Build history of the part. All positions in model axes, mm. Give positions to 0.01 mm unless a question says otherwise; leave off trailing zeros. Write each loop counter-clockwise with the first axis right and the second up, starting at its lowest first coordinate (ties: lowest second). Pieces come first, ordered by that corner, then holes.
from build123d import *

# Parameters (mm, degrees)
SKETCH_1_W      = 72
SKETCH_1_H      = 70
SKETCH_1_R      = 2
SKETCH_1_W_2    = 40
SKETCH_1_H_2    = 40
EXTRUDE_1_DEPTH = 3
CHAMFER_1_SIZE  = 10
CHAMFER_2_SIZE  = 5


with BuildPart() as part:
    # 草图1 → 凸台-拉伸1 (new body)
    with BuildSketch(Plane(origin=(0, 0, 0), x_dir=(1, 0, 0), z_dir=(0, 1, 0))):
        Rectangle(SKETCH_1_W, SKETCH_1_H)
        with Locations(Location((-30, 30, 0), (0, 0, 270))):
            Circle(SKETCH_1_R, mode=Mode.SUBTRACT)
        with Locations(Location((30, 30, 0), (0, 0, 270))):
            Circle(SKETCH_1_R, mode=Mode.SUBTRACT)
        with Locations(Location((30, -30, 0), (0, 0, 270))):
            Circle(SKETCH_1_R, mode=Mode.SUBTRACT)
        with Locations(Location((-30, -30, 0), (0, 0, 270))):
            Circle(SKETCH_1_R, mode=Mode.SUBTRACT)
        Rectangle(SKETCH_1_W_2, SKETCH_1_H_2, mode=Mode.SUBTRACT)
    extrude(amount=EXTRUDE_1_DEPTH)

    # 倒角1
    chamfer_1_edges = [part.edges().sort_by_distance(p)[0] for p in [
        (20, 1.5, -20),
        (-20, 1.5, -20),
        (-20, 1.5, 20),
        (20, 1.5, 20),
    ]]
    chamfer(chamfer_1_edges, length=CHAMFER_1_SIZE)

    # 倒角2
    chamfer_2_edges = [part.edges().sort_by_distance(p)[0] for p in [
        (-36, 1.5, 35),
        (-36, 1.5, -35),
        (36, 1.5, -35),
        (36, 1.5, 35),
    ]]
    chamfer(chamfer_2_edges, length=CHAMFER_2_SIZE)


solid = part.part
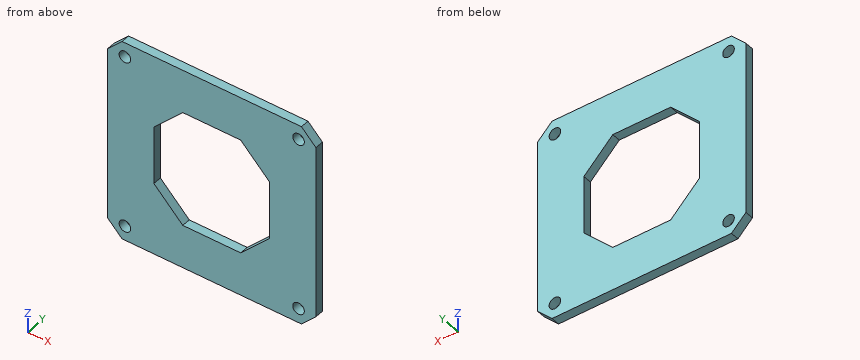
(1) Saw through at B-B, the plane z = 18.5. List the corners of the cut face in (x, y), plus the area to 3 significant figures.
(2) Probe line 1 (X direction, y = 1.8, z = 30); line 2 (X direction, y = 2.4, z = -9.5); line 3 (X direction, y = 2.2, z = 31.5). List the from-to ranges inside material, lowest first.
(3) Saw through at C-C, the plane y = 2.4. List the corners of the cut face in (x, z), plus the area to 3 significant figures.
(4) Drop flat-ended pins along their axis: pin 1 (1 mm diameter, centred on x = 18.5, z = -19.5, fed in from -Y); pin 2 (3.5 mm diameter, centred on x = 30, z = -30, fed in from -Y). Give the stop position or say it passes through.
(5) Saw through at D-D, the plane x = -30. List the corners of the cut face in (y, z), plus the area to 3 significant figures.
(6) Saw through at A-A, the plane x = 17.5. List the corners of the cut face in (y, z).
Computed values:
1. outline: (-36, 0) - (-11.5, 0) - (-11.5, 3) - (-36, 3) - close; (11.5, 0) - (36, 0) - (36, 3) - (11.5, 3) - close
1. area: 147 mm2
2. line 1: x = -36 to -32, -28 to 28, 32 to 36
2. line 2: x = -36 to -20, 20 to 36
2. line 3: x = -34.5 to -31.32, -28.68 to 28.68, 31.32 to 34.5
3. outline: (-36, -30) - (-31, -35) - (31, -35) - (36, -30) - (36, 30) - (31, 35) - (-31, 35) - (-36, 30) - close; hole circle Ø4 at (-30, -30); hole circle Ø4 at (-30, 30); hole (-20, -10) - (-10, -20) - (10, -20) - (20, -10) - (20, 10) - (10, 20) - (-10, 20) - (-20, 10) - close; hole circle Ø4 at (30, -30); hole circle Ø4 at (30, 30)
3. area: 3,540 mm2
4. pin 1: stops at y = 0
4. pin 2: passes through
5. outline: (0, -35) - (3, -35) - (3, -32) - (0, -32) - close; (0, -28) - (3, -28) - (3, 28) - (0, 28) - close; (0, 32) - (3, 32) - (3, 35) - (0, 35) - close
5. area: 186 mm2
6. outline: (0, -35) - (3, -35) - (3, -12.5) - (0, -12.5) - close; (0, 12.5) - (3, 12.5) - (3, 35) - (0, 35) - close
